Work out the finished part from the listing and answer in its coordinate system (mm). Face numbers are marked on the shaded views. Coordinates: 2 decimals unless noted, no trailing zeros. Loops run counter-clockwise (first coordinate to the right, second up) from the corner with the lowest first, then second, coordinate; pieces in that order, holes last. Notation, with made-up numbers: (13.25, 51.5) - (38.25, 51.5) arc R16 ccw to (38.25, 75.5) - close; hole circle Ø3 at (19.25, -20.75). An arc over 180 degrees is marked (long way). Write each question's results on one line, items separated by ' | '. Start each with the question number.
1. Find the intervals of material crossed by line 1 along Z through (x, y) = (170, 0.25); line 2 along Z through (x, y) = (80.5, 5); line 3 along Z through (x, y) = (126, 1.25), in increasing order. Write a range as [from, to].
2. Determine the mould class of the marked faces 1 and 2 for opening direction Z: released by +Z, released by -Z, zero draft, split by the parting line, or undercut.
3. A cutting plane is placed at C-C on x = 97. Determine the outline of the cut face in (y, z), then the cut area to 3 significant figures.
4. A cutting plane is placed at D-D on z = -57.5. Determine the outline of the cut face in (x, y), then the cut area to 3 significant figures.
5. Each of these flat-tipped pins is pushed along its axis until it touches: P1, Ø1, axis at y = -1.5, z = -78, coming from the +X side; P2, Ø5, axis at y = 2.5, z = -86, coming from the +X side; P3, Ø5, axis at y = 3, z = -109, coming from the +X side. Where does it stop, or does it pass through?
6. A cutting plane is placed at A-A on x = 170. Determine the outline of the cut face in (y, z), then the cut area to 3 significant figures.
7. A cutting plane is placed at B-B on y = -2.25. Determine the outline of the cut face in (x, z).
from build123d import *

# Parameters (mm, degrees)
SKETCH1_W           = 190
SKETCH1_H           = 160
BOSS_EXTRUDE1_DEPTH = 6
CUT_EXTRUDE1_DEPTH  = 10
SKETCH3_W           = 185
SKETCH3_H           = 4
SKETCH3_W_2         = 5
SKETCH3_H_2         = 152
BOSS_EXTRUDE3_DEPTH = 4
SKETCH4_R           = 4.5
CUT_EXTRUDE2_DEPTH  = 5
SKETCH5_R           = 3
CUT_EXTRUDE7_DEPTH  = 5


with BuildPart() as part:
    # Sketch1 → Boss-Extrude1 (new body)
    with BuildSketch(Plane(origin=(0, 0, 0), x_dir=(1, 0, 0), z_dir=(0, 1, 0))):
        with Locations((95, 80)):
            Rectangle(SKETCH1_W, SKETCH1_H)
    extrude(amount=BOSS_EXTRUDE1_DEPTH)

    # Sketch2 → Cut-Extrude1 (cut)
    with BuildSketch(Plane(origin=(0, 6, 0), x_dir=(1, 0, 0), z_dir=(0, 1, 0))):
        with BuildLine():
            ThreePointArc((34.503849117, 8.335899411), (38.664100589, 7.503849117), (39.496150883, 11.664100589))
            Line((39.496150883, 11.664100589), (20.605551275, 40))
            Line((20.605551275, 40), (19.496150883, 41.664100589))
            ThreePointArc((19.496150883, 41.664100589), (15.335899411, 42.496150883), (14.503849117, 38.335899411))
            Line((14.503849117, 38.335899411), (34.503849117, 8.335899411))
        make_face()
        with BuildLine():
            Line((10, 100), (10, 60))
            ThreePointArc((10, 60), (12.928932188, 52.928932188), (20, 50))
            Line((20, 50), (100, 50))
            ThreePointArc((100, 50), (104.617486132, 48.870108332), (108.191520443, 45.735764364))
            Line((108.191520443, 45.735764364), (116.223971332, 34.264235636))
            ThreePointArc((116.223971332, 34.264235636), (119.798005643, 31.129891668), (124.415491775, 30))
            Line((124.415491775, 30), (190, 30))
            Line((190, 30), (190, 130))
            Line((190, 130), (124.415491775, 130))
            ThreePointArc((124.415491775, 130), (119.798005643, 128.870108332), (116.223971332, 125.735764364))
            Line((116.223971332, 125.735764364), (108.191520443, 114.264235636))
            ThreePointArc((108.191520443, 114.264235636), (104.617486132, 111.129891668), (100, 110))
            Line((100, 110), (20, 110))
            ThreePointArc((20, 110), (12.928932188, 107.071067812), (10, 100))
        make_face()
        with BuildLine():
            Line((34.503849117, 38.335899411), (54.503849117, 8.335899411))
            ThreePointArc((54.503849117, 8.335899411), (58.664100589, 7.503849117), (59.496150883, 11.664100589))
            Line((59.496150883, 11.664100589), (39.496150883, 41.664100589))
            ThreePointArc((39.496150883, 41.664100589), (35.335899411, 42.496150883), (34.503849117, 38.335899411))
        make_face()
        with BuildLine():
            Line((54.503849117, 38.335899411), (74.503849117, 8.335899411))
            ThreePointArc((74.503849117, 8.335899411), (78.664100589, 7.503849117), (79.496150883, 11.664100589))
            Line((79.496150883, 11.664100589), (59.496150883, 41.664100589))
            ThreePointArc((59.496150883, 41.664100589), (55.335899411, 42.496150883), (54.503849117, 38.335899411))
        make_face()
        with BuildLine():
            Line((74.503849117, 38.335899411), (94.503849117, 8.335899411))
            ThreePointArc((94.503849117, 8.335899411), (98.664100589, 7.503849117), (99.496150883, 11.664100589))
            Line((99.496150883, 11.664100589), (79.496150883, 41.664100589))
            ThreePointArc((79.496150883, 41.664100589), (75.335899411, 42.496150883), (74.503849117, 38.335899411))
        make_face()
        with BuildLine():
            Line((94.503849117, 38.335899411), (113.394448725, 10))
            Line((113.394448725, 10), (114.503849117, 8.335899411))
            ThreePointArc((114.503849117, 8.335899411), (118.664100589, 7.503849117), (119.496150883, 11.664100589))
            Line((119.496150883, 11.664100589), (99.496150883, 41.664100589))
            ThreePointArc((99.496150883, 41.664100589), (96.130647554, 42.871276079), (94, 40))
            ThreePointArc((94, 40), (94.128723921, 39.130647554), (94.503849117, 38.335899411))
        make_face()
        with BuildLine():
            ThreePointArc((94.503849117, 121.664100589), (95.335899411, 117.503849117), (99.496150883, 118.335899411))
            Line((99.496150883, 118.335899411), (119.496150883, 148.335899411))
            ThreePointArc((119.496150883, 148.335899411), (118.664100589, 152.496150883), (114.503849117, 151.664100589))
            Line((114.503849117, 151.664100589), (94.503849117, 121.664100589))
        make_face()
        with BuildLine():
            ThreePointArc((74.503849117, 121.664100589), (75.335899411, 117.503849117), (79.496150883, 118.335899411))
            Line((79.496150883, 118.335899411), (99.496150883, 148.335899411))
            ThreePointArc((99.496150883, 148.335899411), (98.664100589, 152.496150883), (94.503849117, 151.664100589))
            Line((94.503849117, 151.664100589), (74.503849117, 121.664100589))
        make_face()
        with BuildLine():
            ThreePointArc((54.503849117, 121.664100589), (55.335899411, 117.503849117), (59.496150883, 118.335899411))
            Line((59.496150883, 118.335899411), (79.496150883, 148.335899411))
            ThreePointArc((79.496150883, 148.335899411), (78.664100589, 152.496150883), (74.503849117, 151.664100589))
            Line((74.503849117, 151.664100589), (54.503849117, 121.664100589))
        make_face()
        with BuildLine():
            ThreePointArc((34.503849117, 121.664100589), (35.335899411, 117.503849117), (39.496150883, 118.335899411))
            Line((39.496150883, 118.335899411), (59.496150883, 148.335899411))
            ThreePointArc((59.496150883, 148.335899411), (58.664100589, 152.496150883), (54.503849117, 151.664100589))
            Line((54.503849117, 151.664100589), (34.503849117, 121.664100589))
        make_face()
        with BuildLine():
            ThreePointArc((14.503849117, 121.664100589), (15.335899411, 117.503849117), (19.496150883, 118.335899411))
            Line((19.496150883, 118.335899411), (39.496150883, 148.335899411))
            ThreePointArc((39.496150883, 148.335899411), (38.664100589, 152.496150883), (34.503849117, 151.664100589))
            Line((34.503849117, 151.664100589), (14.503849117, 121.664100589))
        make_face()
    extrude(amount=-CUT_EXTRUDE1_DEPTH, mode=Mode.SUBTRACT)

    # Sketch3 → Boss-Extrude3 (add)
    with BuildSketch(Plane.XZ):
        with Locations((97.5, -158)):
            Rectangle(SKETCH3_W, SKETCH3_H)
        with Locations((2.5, -158)):
            Rectangle(SKETCH3_W_2, SKETCH3_H)
        with Locations((2.5, -80)):
            Rectangle(SKETCH3_W_2, SKETCH3_H_2)
        with Locations((97.5, -2)):
            Rectangle(SKETCH3_W, SKETCH3_H)
        with Locations((2.5, -2)):
            Rectangle(SKETCH3_W_2, SKETCH3_H)
    extrude(amount=BOSS_EXTRUDE3_DEPTH)

    # Sketch4 → Cut-Extrude2 (cut)
    with BuildSketch(Plane(origin=(0, 6, 0), x_dir=(1, 0, 0), z_dir=(0, 1, 0))):
        with Locations(Location((170, 140, 0), (0, 0, 270))):
            Circle(SKETCH4_R)
        with Locations(Location((40, 140, 0), (0, 0, 270))):
            Circle(SKETCH4_R)
        with Locations(Location((170, 20, 0), (0, 0, 90))):
            Circle(SKETCH4_R)
        with Locations(Location((40, 20, 0), (0, 0, 90))):
            Circle(SKETCH4_R)
    extrude(amount=-CUT_EXTRUDE2_DEPTH, mode=Mode.SUBTRACT)

    # Sketch5 → Cut-Extrude7 (cut)
    with BuildSketch(Plane(origin=(0, 0, 0), x_dir=(1, 0, 0), z_dir=(0, 1, 0))):
        with Locations(Location((170, 140, 0), (0, 0, 270))):
            Circle(SKETCH5_R)
        with Locations(Location((40, 140, 0), (0, 0, 270))):
            Circle(SKETCH5_R)
        with Locations(Location((170, 20, 0), (0, 0, 90))):
            Circle(SKETCH5_R)
        with Locations(Location((40, 20, 0), (0, 0, 90))):
            Circle(SKETCH5_R)
    extrude(amount=CUT_EXTRUDE7_DEPTH, mode=Mode.SUBTRACT)


solid = part.part
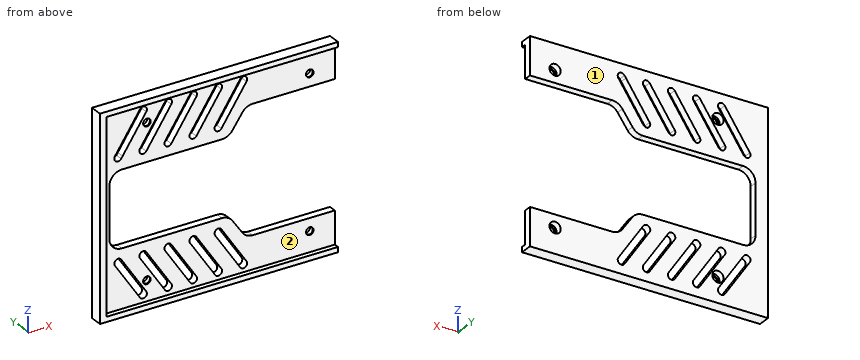
Values:
1) line 1: [-160, -143], [-137, -130], [-30, -23], [-17, 0] | line 2: [-160, -130.66], [-119.84, -110], [-50, -40.16], [-29.34, 0] | line 3: [-160, -130], [-30, 0]
2) face 1: zero draft | face 2: undercut
3) outline: (-4, -160) - (6, -160) - (6, -153) - (0, -153) - (0, -156) - (-4, -156) - close; (-4, -4) - (0, -4) - (0, -7) - (6, -7) - (6, 0) - (-4, 0) - close; (0, -144.59) - (6, -144.59) - (6, -125.41) - (0, -125.41) - close; (0, -117) - (6, -117) - (6, -110) - (0, -110) - close; (0, -50) - (6, -50) - (6, -43) - (0, -43) - close; (0, -34.59) - (6, -34.59) - (6, -15.41) - (0, -15.41) - close | area: 430 mm^2
4) outline: (0, -4) - (5, -4) - (5, 0) - (10.32, 0) - (10.32, 6) - (0, 6) - close | area: 81.9 mm^2
5) P1: x = 5 | P2: x = 10 | P3: x = 105.27
6) outline: (-4, -160) - (6, -160) - (6, -144.5) - (1, -144.5) - (1, -143) - (0, -143) - (0, -156) - (-4, -156) - close; (-4, -4) - (0, -4) - (0, -17) - (1, -17) - (1, -15.5) - (6, -15.5) - (6, 0) - (-4, 0) - close; (0, -137) - (1, -137) - (1, -135.5) - (6, -135.5) - (6, -130) - (0, -130) - close; (0, -30) - (6, -30) - (6, -24.5) - (1, -24.5) - (1, -23) - (0, -23) - close | area: 290 mm^2
7) outline: (0, -160) - (190, -160) - (190, -156) - (5, -156) - (5, -4) - (190, -4) - (190, 0) - (0, 0) - close
